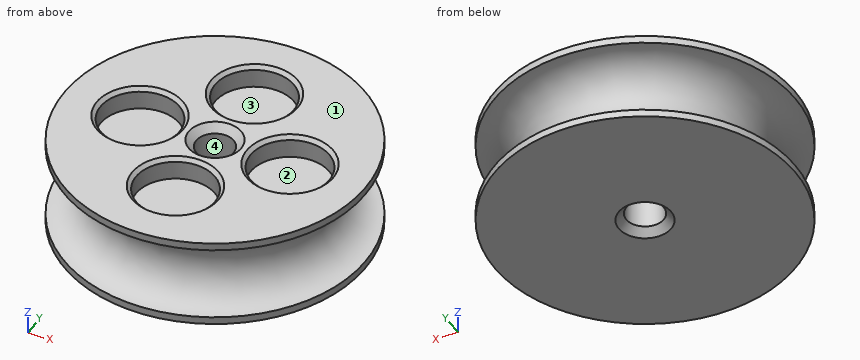
from build123d import *

# Parameters (mm, degrees)
TORUS_R         = 5
SKETCH_R        = 20
PAD_DEPTH       = 12
SKETCH001_R     = 2.5
POCKET_DEPTH    = 12
SKETCH002_R     = 5.25
POCKET001_DEPTH = 3
CHAMFER_SIZE    = 0.5
CHAMFER001_SIZE = 1


with BuildPart() as torus:
    # Torus → Torus (revolve)
    with BuildSketch(Plane(origin=(0, 0, 6), x_dir=(1, 0, 0), z_dir=(0, -1, 0))):
        with Locations((20, 0)):
            Circle(TORUS_R)
    revolve(axis=Axis((0, 0, 6), (0, 0, 1)))


with BuildPart() as cut:
    # Sketch → Pad (new body)
    with BuildSketch(Plane.XY):
        Circle(SKETCH_R)
    extrude(amount=PAD_DEPTH)

    # Sketch001 (on Face3 of Pad) → Pocket (cut)
    with BuildSketch(Plane.XY.offset(12)):
        Circle(SKETCH001_R)
    extrude(amount=-POCKET_DEPTH, mode=Mode.SUBTRACT)

    # Sketch002 (on Face3 of Pocket) → Pocket001 (cut)
    with BuildSketch(Plane.XY.offset(12)):
        with Locations((-10, 0)):
            Circle(SKETCH002_R)
        with Locations((10, 0)):
            Circle(SKETCH002_R)
        with Locations((0, 10)):
            Circle(SKETCH002_R)
        with Locations((0, -10)):
            Circle(SKETCH002_R)
    extrude(amount=-POCKET001_DEPTH, mode=Mode.SUBTRACT)

    # Chamfer
    chamfer_edges = [cut.edges().sort_by_distance(p)[0] for p in [
        (-5.25, 10, 12),
        (-15.25, 0, 12),
        (-5.25, -10, 12),
        (4.75, 0, 12),
    ]]
    chamfer(chamfer_edges, length=CHAMFER_SIZE)

    # Chamfer001
    chamfer001_edges = [cut.edges().sort_by_distance(p)[0] for p in [
        (-2.5, 0, 12),
        (-2.5, 0, 0),
    ]]
    chamfer(chamfer001_edges, length=CHAMFER001_SIZE)

    # Cut: cut Torus
    add(torus.part, mode=Mode.SUBTRACT)


solid = cut.part
Read the model definition and answer for the solid it produces. Units are mm, in the model's axes. Face numbers are marked on the shaded views. A direction names the side the tool comes from. Give positions to 0.01 mm unless a question says otherwise; leave off trailing zeros. Loops run counter-clockwise (first coordinate to the right, second up) from the corner with the lowest first, then second, coordinate; pieces in that order, holes last. Notation, with made-up numbers: (83.5, 80) - (88.5, 80) arc R5 cw to (88.5, 88) - close; hole circle Ø9 at (37, 50.5). An arc over 180 degrees is marked (long way). Answer as CSV lines item,"result". Start each with the question number.
1) Find section A-A (y = 0). Write down the section's boundary in (x, z), then the cut area to 3 significant figures.
2) Each of these flat-tipped pins is pushed along its axis until it touches: pin 1 Ø2 at (x, z) = (-3.5, 8) entering from -Y; pin 2 Ø5 at (x, z) = (-14, 4.5) entering from -Y; pin 3 Ø3 at (x, z) = (-6, 6) entering from -Y. Where does it stop, or does it pass through?
3) Determine the mould class of the marked faces 1 and 2 for opening direction Y: released by +Y, released by -Y, zero draft, split by the parting line, or undercut.
4) Find section C-C (z = 7.5). Write down the section's boundary in (x, y).
5) Straight lines are drawn through the part: L1, parallel to Y at x = -1.5, z = 10.25; L2, parallel to Y at x = -4.5, z = 9.25; L3, parallel to X at y = -3, z = 9.25. For each, find the intervals that lie inside material, in ascending order. Write a range as from..to.
6) Which of the six approach directions +Z, -Z, +X, -X, +Y, -Y give full straight-line access (tool end or side, diameter ignored) to the marked faces 3 and 4?
7) Find section B-B (z = 2). Write down the section's boundary in (x, y), then the cut area to 3 significant figures.
Findings below:
1,outline,"(-20, 0) - (-3.5, 0) - (-2.5, 1) - (-2.5, 11) - (-3.5, 12) - (-4.25, 12) - (-4.75, 11.5) - (-4.75, 9) - (-15.25, 9) - (-15.25, 11.5) - (-15.75, 12) - (-20, 12) - (-20, 11) arc R5 cw to (-20, 1) - close; (2.5, 1) - (3.5, 0) - (20, 0) - (20, 1) arc R5 cw to (20, 11) - (20, 12) - (15.75, 12) - (15.25, 11.5) - (15.25, 9) - (4.75, 9) - (4.75, 11.5) - (4.25, 12) - (3.5, 12) - (2.5, 11) - close"
1,area,"276 mm^2"
2,pin 1,"y = -15.64"
2,pin 2,"y = -10.66"
2,pin 3,"y = -14.31"
3,face 1,"zero draft"
3,face 2,"undercut"
4,outline,"circle Ø30.46 at (0, 0); hole circle Ø5 at (0, 0)"
5,L1,"-17.3..-15.03, -4.97..-2, 2..4.97, 15.03..17.3"
5,L2,"-15.56..-12.7, -7.3..7.3, 12.7..15.56"
5,L3,"-15.92..-14.31, -5.69..5.69, 14.31..15.92"
6,face 3,"+Z"
6,face 4,"+Z, -Z"
7,outline,"circle Ø34 at (0, 0); hole circle Ø5 at (0, 0)"
7,area,"888 mm^2"
